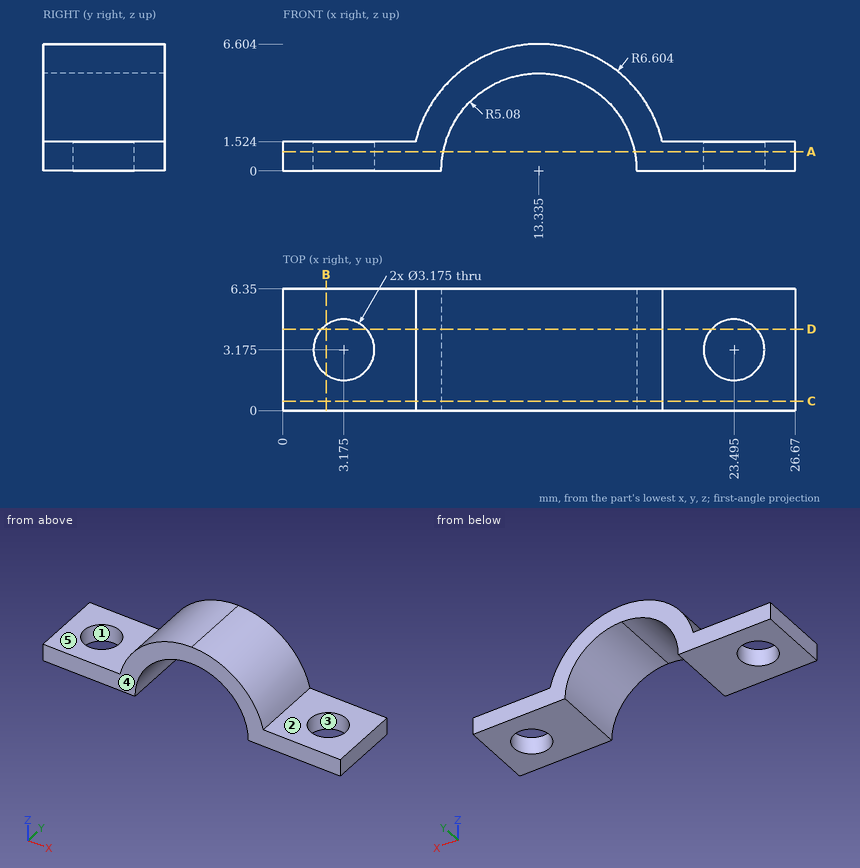
Part print with two shaded views. Sizes in mm from the minimum x, y, z corner. A direction names the side the tool comes from. Round coordinates to 2 decimals unless told otherwise and drop trailing zeros. Loops run counter-clockwise (first coordinate to the right, second up) from the corner with the lowest first, then second, coordinate; pieces in that order, holes last.
Item 1: Which spindle directions (+Z, -Z, +X, -X, +Y, -Y) get a long thin tool onto all of the face, cutting with end or side? Do the marked faces 4 and 5. Say none if no direction does.
Item 2: Two-plate mould, pull along X, no slides. Class the marked faces 1, 2 and 3: released by +X, released by -X, zero draft, split by the parting line, or undercut.
Item 3: Drill centre lines: line 1 along Z through (x, y) = (23, 5.5); line 2 along X through (y, z) = (3.75, 0.75); line 3 along X through (y, z) = (2.75, 3.25). Where is each one in solid material? Low to high.
Item 4: Pin check, flat tips, straight feed: P1, Ø2, axis at x = 17, z = 3, coming from the -Y side; P2, Ø1.9, axis at x = 22.5, y = 4, coming from the +Z side; P3, Ø1, axis at y = 3, z = 4.5, coming from the -X side; P4, Ø2, axis at y = 1, z = 4.5, coming from the -X side. Stop position of each tip, or through.
Item 5: Saw through at C-C (y = 0.5). List the corners of the cut face in (x, z) (3 decimals).
Item 6: Saw through at B-B (x = 2.25). List the corners of the cut face in (y, z).
Item 7: Saw through at D-D (y = 4.25). List the corners of the cut face in (x, z) (3 decimals).
Item 8: Saw through at A-A (z = 1). State how many separate pieces and enclosed holes the cut face has, then the cut area to 3 significant figures.
Worked answers:
1. face 4: +Z, -Z, +X, -X, -Y
1. face 5: +Z, -X, +Y, -Y
2. face 1: undercut
2. face 2: zero draft
2. face 3: undercut
3. line 1: z = 0 to 1.52
3. line 2: x = 0 to 1.7, 4.65 to 8.31, 18.36 to 22.02, 24.97 to 26.67
3. line 3: x = 7.59 to 9.43, 17.24 to 19.08
4. P1: stops at y = 0
4. P2: stops at z = 1.52
4. P3: stops at x = 8.08
4. P4: stops at x = 7.73
5. outline: (0, 0) - (8.255, 0) arc R5.08 cw to (13.335, 5.08) arc R5.08 cw to (18.415, 0) - (26.67, 0) - (26.67, 1.524) - (19.761, 1.524) arc R6.604 ccw to (13.335, 6.604) arc R6.604 ccw to (6.909, 1.524) - (0, 1.524) - close
6. outline: (0, 0) - (1.88, 0) - (1.88, 1.52) - (0, 1.52) - close; (4.47, 0) - (6.35, 0) - (6.35, 1.52) - (4.47, 1.52) - close
7. outline: (0, 0) - (2.007, 0) - (2.007, 1.524) - (0, 1.524) - close; (4.343, 0) - (8.255, 0) arc R5.08 cw to (13.335, 5.08) arc R5.08 cw to (18.415, 0) - (22.327, 0) - (22.327, 1.524) - (19.761, 1.524) arc R6.604 ccw to (13.335, 6.604) arc R6.604 ccw to (6.909, 1.524) - (4.343, 1.524) - close; (24.663, 0) - (26.67, 0) - (26.67, 1.524) - (24.663, 1.524) - close
8. separate pieces: 2
8. enclosed holes: 2
8. area: 90.3 mm2
